from build123d import *

# Parameters (mm, degrees)
BOSS_EXTRUDE1_DEPTH     = 504
CUT_EXTRUDE2_REACH      = 516.263
CUT_EXTRUDE2_END_RADIUS = 90
SKETCH3_R               = 2.5
CUT_EXTRUDE3_REACH      = 516.263
CUT_EXTRUDE3_END_RADIUS = 90
SKETCH5_R               = 2.5
LPATTERN2_COUNT         = 2
LPATTERN2_PITCH         = 491


with BuildPart() as part:
    # Sketch1 → Boss-Extrude1 (new body)
    with BuildSketch(Plane(origin=(0, 0, 0), x_dir=(1, 0, 0), z_dir=(0, 1, 0))):
        with BuildLine():
            Line((0, 92), (0, 90))
            ThreePointArc((0, 90), (63.639610307, 63.639610307), (90, 0))
            Line((90, 0), (92, 0))
            ThreePointArc((92, 0), (65.053823869, 65.053823869), (0, 92))
        make_face()
    extrude(amount=BOSS_EXTRUDE1_DEPTH)

    # Cut-Extrude2: up to this cylinder (the profile starts outside it)
    cut_extrude2_end = Plane(origin=(0, 6.5, 0), z_dir=(0, -1, 0)) * Cylinder(CUT_EXTRUDE2_END_RADIUS, 1213.526, mode=Mode.PRIVATE)
    # Sketch3 → Cut-Extrude2 (cut, up to the surface)
    with BuildSketch(Plane(origin=(84.996916991, 0, -35.206875778), x_dir=(-0.38268343236509045, 0, -0.9238795325112865), z_dir=(0.9238795325112865, 0, -0.38268343236509045)), mode=Mode.PRIVATE) as cut_extrude2_sk1:
        with Locations((0, 6.5)):
            Circle(SKETCH3_R)
    cut_extrude2_tool1 = extrude(cut_extrude2_sk1.sketch, amount=-CUT_EXTRUDE2_REACH, mode=Mode.PRIVATE) - cut_extrude2_end
    cut_extrude2 = cut_extrude2_tool1.solids().sort_by_distance((84.996917, 6.5, -35.206876))[0]
    add(cut_extrude2, mode=Mode.SUBTRACT)

    # Cut-Extrude3: up to this cylinder (the profile starts outside it)
    cut_extrude3_end = Plane(origin=(0, 6.5, 0), z_dir=(0, -1, 0)) * Cylinder(CUT_EXTRUDE3_END_RADIUS, 1213.526, mode=Mode.PRIVATE)
    # Sketch5 → Cut-Extrude3 (cut, up to the surface)
    with BuildSketch(Plane(origin=(35.206875778, 0, -84.996916991), x_dir=(-0.9238795325112878, 0, -0.3826834323650876), z_dir=(0.3826834323650876, 0, -0.9238795325112878)), mode=Mode.PRIVATE) as cut_extrude3_sk1:
        with Locations((0, 6.5)):
            Circle(SKETCH5_R)
    cut_extrude3_tool1 = extrude(cut_extrude3_sk1.sketch, amount=-CUT_EXTRUDE3_REACH, mode=Mode.PRIVATE) - cut_extrude3_end
    cut_extrude3 = cut_extrude3_tool1.solids().sort_by_distance((35.206876, 6.5, -84.996917))[0]
    add(cut_extrude3, mode=Mode.SUBTRACT)

    # LPattern2: Cut-Extrude2, Cut-Extrude3 ×2
    with Locations(*[(0, i * LPATTERN2_PITCH, 0) for i in range(1, LPATTERN2_COUNT)]):
        add(cut_extrude2, mode=Mode.SUBTRACT)
        add(cut_extrude3, mode=Mode.SUBTRACT)


solid = part.part
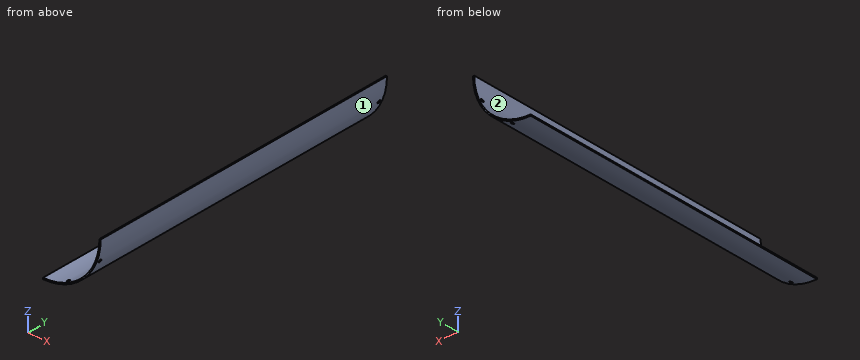
Here's how the part is built. I have some questions about the finished solid (model axes, mm). Face numbers are marked on the shaded views. Round coordinates to 2 decimals unless told otherwise and drop trailing zeros. Write each loop counter-clockwise with the first axis right and the second up, starting at its lowest first coordinate (ties: lowest second). Pieces come first, ordered by that corner, then holes.
1. I need wall thicknesses on L1, parallel to X at y = 394, z = -35.5; L2, parallel to X at y = 352, z = -19.5; L3, parallel to Z at x = 65, y = 266.5. Which ranges of each line are inside material? Lowest first, please.
2. Suppose I cut it at A-A (y = 205). List the corners of the cut face in (x, z) for me.
3. Will these pins go through, and if not, where does the flat tip stop? pin 1 Ø8 at (x, y) = (36, 291) entering from +Z; pin 2 Ø12 at (x, y) = (39.5, 406) entering from +Z; pin 3 Ø12 at (y, z) = (222.5, -24) entering from -X.
4. If we mould it in two halves opening along X, with no side actions, what happens to the marked faces 1 and 2? For each: released by +X, released by -X, zero draft, split by the parting line, or undercut.
5. Suppose I cut it at B-B (x = 11). List the corners of the cut face in (y, z) for me.
Answer sheet:
1. L1: x = 82.7 to 84.87
1. L2: x = 87.86 to 89.91
1. L3: z = -65.11 to -62.25
2. outline: (0, -92) arc R92 ccw to (92, 0) - (90, 0) arc R90 cw to (0, -90) - close
3. pin 1: stops at z = -80.62
3. pin 2: stops at z = -77.65
3. pin 3: stops at x = 84.85
4. face 1: released by +X
4. face 2: released by -X
5. outline: (0, -91.34) - (504, -91.34) - (504, -89.33) - (0, -89.33) - close
